Design review of the part built by this model. Coordinates are the model's own, in mm. A direction names the side the tool comes from. Round coordinates to 2 decimals unless told otherwise and drop trailing zeros. Order: outer loops, then holes, each group sorted by start corner. A loop starts at its lowest first (then second) coordinate and runs counter-clockwise, first axis right, second up. Notation, with made-up numbers: M 56,23 L 106,23 A30 ccw 106,52 Z; hole C 0.5,33 d10. An arc over 180 degrees is marked long. Use a Markdown table: item, result. Add a question column.
(1) For pin 1 (12.5 mm diameter, centred on x = -55, z = 29, fed in from +Y); pin 2 (0.9 mm diameter, centred on y = 1, z = -13.5, fed in from -X); pin 3 (9 mm diameter, centred on x = 55, z = -29, fed in from -Y); pin 4 (11 mm diameter, centred on x = 39.5, z = 1, fed in from -Y), all flat-tipped, find the tip position at first contact; note any pin that passes through.
(2) Machinability: for faces 1 (the face through (49, 3, 1)), 2 (the face through (49.505, 9.409, 29.242)), 3 (the face through (-22, 15, 1)), 4 (the face through (44, 16, 1)), 5 (the face through (-30, 1, 1)), which of the approach directions +Z, -Z, +X, -X, +Y, -Y give a long, thin tool a straight path to every point of the face, cutting with its end or side? Answer none if there is none.
(3) To check wall thickness, follow probe 1 along Z at (x, y) = (55, 7.5); probe 2 along X at (y, z) = (6.75, -25); probe 3 along Y at (x, z) = (5, -11). State the ranges of each line that lie inside material, in increasing order. Write a range as from..to.
(4) Take a section at B-B (z = 22). Write out the cut boundary in (x, y), then the cut area to 3 significant figures.
(5) The part is to be moulded in two halves that separate along Z. For faces 6 (the face through (49.505, 9.409, -28.758)), 7 (the face through (0, 13, 1)), 8 (the face through (63.58, 9.41, -37.39)), say which applies: released by +Z, released by -Z, zero draft, split by the parting line, or undercut.
(6) Take a section at C-C (x = -47.5). Write out the cut boundary in (y, z).
(7) Take a section at D-D (y = 1.5). Write out the cut boundary in (x, z).
(8) Take a section at A-A (y = 11.25). Write out the cut boundary in (x, z), then the cut area to 3 significant figures.
```python
from build123d import *

# Parameters (mm, degrees)
EXTRUSION1_DEPTH   = 41
CONG_1_R           = 12
D_GAGEMENT_M1_61_D = 11


with BuildPart() as part:
    # Esquisse1 → Extrusion1 (new, symmetric)
    with BuildSketch(Plane.XY):
        Polygon((22, 16), (67, 16), (67, 3), (30, 3), (30, 0), (-30, 0), (-30, 3), (-67, 3), (-67, 16), (-22, 16), (-22, 13), (22, 13), align=None)
    extrude(amount=EXTRUSION1_DEPTH, both=True)

    # Congé1
    cong_1_edges = [part.edges().sort_by_distance(p)[0] for p in [
        (67, 9.5, -41),
        (-67, 9.5, -41),
        (67, 9.5, 41),
        (-67, 9.5, 41),
    ]]
    fillet(cong_1_edges, radius=CONG_1_R)

    # Dégagement M1.61 (through all)
    with Locations(Plane(origin=(0, 16, 0), x_dir=(-1, 0, 0), z_dir=(0, 1, 0))):
        with Locations((55, 29), (55, -29), (-55, -29), (-55, 29)):
            Hole(D_GAGEMENT_M1_61_D / 2)


solid = part.part
```
Verdict:
| question | item | result |
|---|---|---|
| 1 | pin 1 | stops at y = 16 |
| 1 | pin 2 | stops at x = -30 |
| 1 | pin 3 | passes through |
| 1 | pin 4 | stops at y = 3 |
| 2 | face 1 | +Z, -Z, +X, -Y |
| 2 | face 2 | +Y, -Y |
| 2 | face 3 | +Z, -Z, +Y |
| 2 | face 4 | +Z, -Z, +X, -X, +Y |
| 2 | face 5 | +Z, -Z, -X, -Y |
| 3 | probe 1 | z = -41..-34.5, -23.5..23.5, 34.5..41 |
| 3 | probe 2 | x = -67..-58.77, -51.23..51.23, 58.77..67 |
| 3 | probe 3 | y = 0..13 |
| 4 | outline | M -67,3 L -30,3 L -30,0 L 30,0 L 30,3 L 67,3 L 67,16 L 22,16 L 22,13 L -22,13 L -22,16 L -67,16 Z |
| 4 | area | 1,790 mm^2 |
| 5 | face 6 | undercut |
| 5 | face 7 | zero draft |
| 5 | face 8 | released by -Z |
| 6 | outline | M 3,-41 L 16,-41 L 16,41 L 3,41 Z |
| 7 | outline | M -30,-41 L 30,-41 L 30,41 L -30,41 Z |
| 8 | outline | M -67,-29 A12 ccw -55,-41 L 55,-41 A12 ccw 67,-29 L 67,29 A12 ccw 55,41 L -55,41 A12 ccw -67,29 Z; hole C -55,-29 d11; hole C -55,29 d11; hole C 55,-29 d11; hole C 55,29 d11 |
| 8 | area | 10,500 mm^2 |
